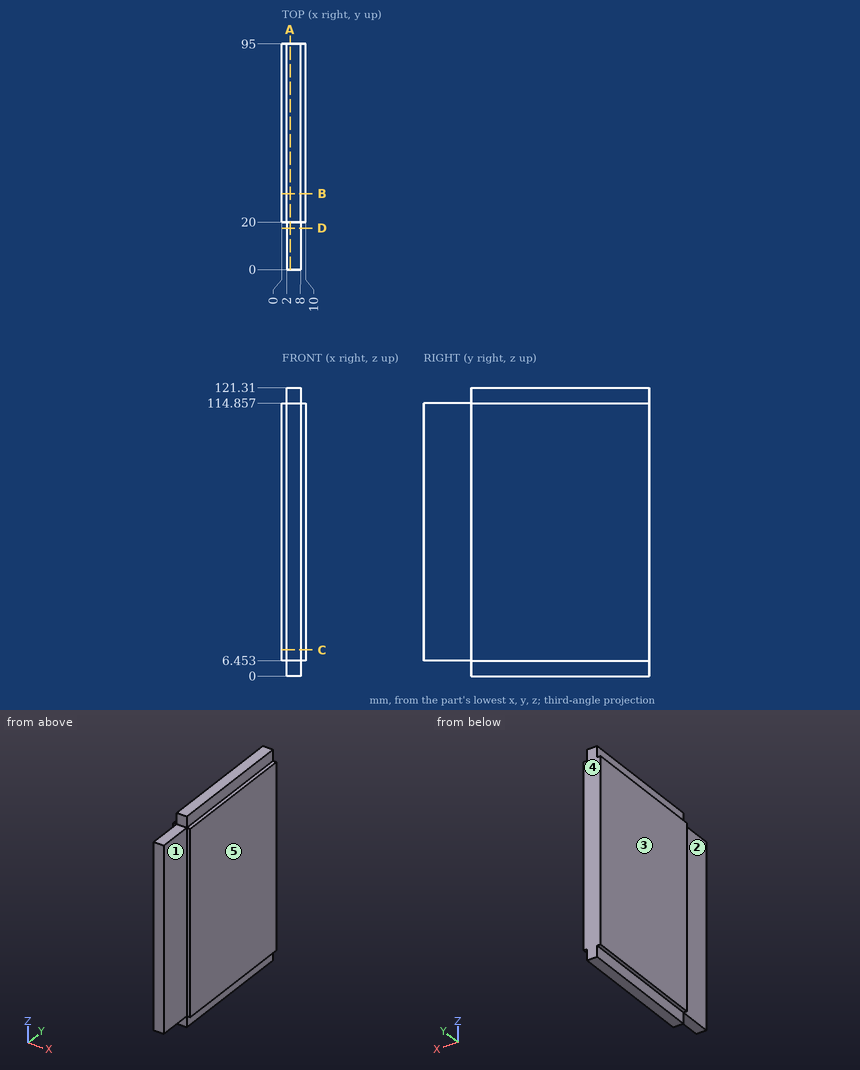
Study the drawing (mm; zero at the part's minimum x, y, z) and answer. A direction names the side the tool comes from. Give positions to 0.01 mm unless a question says otherwise; leave off trailing zeros. Loops run counter-clockwise (first coordinate to the right, second up) from the corner with the lowest first, then second, coordinate; pieces in that order, holes last. Notation, with made-up numbers: (63, 81) - (88, 81) arc R27 cw to (88, 99) - close; hole circle Ø11 at (29.5, 79). An arc over 180 degrees is marked (long way). Return JSON: item names as keys, results as strings. Group by question number.
1. Given pin 1 Ø22 at (y, z) = (8.5, 72.5) entering from +X; pin 2 Ø1 at (x, y) = (9, 50) entering from +Z; pin 3 Ø1.6 at (x, y) = (9.5, 73) entering from -Z, each flat-ended and moving along its own axis, determine where each tip first touches the part or whether it passes through.
2. Which of the six approach directions +Z, -Z, +X, -X, +Y, -Y give full straight-line access (tool end or side, diameter ignored) to the marked faces 1 and 2?
3. Find section D-D (y = 17.5). Write down the section's boundary in (x, z), then the cut area to 3 significant figures.
4. Find section C-C (z = 11). Write down the section's boundary in (x, y).
5. Straight lines are drawn through the part: line 1 (Y direction, x = 0.5, z = 56); line 2 (X direction, y = 15.5, z = 14); line 3 (Z direction, x = 9.5, y = 82). For each, find the intervals that lie inside material, in ascending order. Write a range as [from, to].
6. Determine the mould class of the marked faces 3, 4 and 5 for opening direction X: pulls with the +X half, pulls with the -X half, needs draft (parallel to the pull), parting line crosses it, or undercut.
7. Find section A-A (x = 3.5). Write down the section's boundary in (y, z), then the cut area to 3 significant figures.
8. Find section B-B (y = 32). Write down the section's boundary in (x, z).
Verdict:
{
 "1": {"pin 1": "stops at x = 8", "pin 2": "stops at z = 114.86", "pin 3": "stops at z = 6.45"},
 "2": {"face 1": "+Z, -Z, +X, -Y", "face 2": "+Z, -Z, -X, -Y"},
 "3": {"outline": "(2, 6.45) - (8, 6.45) - (8, 114.86) - (2, 114.86) - close", "area": "650 mm^2"},
 "4": {"outline": "(0, 20) - (2, 20) - (2, 0) - (8, 0) - (8, 20) - (10, 20) - (10, 95) - (0, 95) - close"},
 "5": {"line 1": "y = [20, 95]", "line 2": "x = [2, 8]", "line 3": "z = [6.45, 114.86]"},
 "6": {"face 3": "pulls with the -X half", "face 4": "needs draft", "face 5": "pulls with the +X half"},
 "7": {"outline": "(0, 6.45) - (20, 6.45) - (20, 0) - (95, 0) - (95, 121.31) - (20, 121.31) - (20, 114.86) - (0, 114.86) - close", "area": "11,300 mm^2"},
 "8": {"outline": "(0, 6.45) - (2, 6.45) - (2, 0) - (8, 0) - (8, 6.45) - (10, 6.45) - (10, 114.86) - (8, 114.86) - (8, 121.31) - (2, 121.31) - (2, 114.86) - (0, 114.86) - close"}
}
